CAD build for the part. Positions are in the model's coordinates, mm. A direction names the side the tool comes from. Give positions to 0.01 mm unless a question says otherwise; leave off trailing zeros. Order: outer loops, then holes, each group sorted by start corner. A loop starts at its lowest first (then second) coordinate and runs counter-clockwise, first axis right, second up.
from build123d import *

# Parameters (mm, degrees)
SALIENTE_EXTRUIR1_DEPTH    = 131.1
CROQUIS3_R                 = 1.1
CORTAR_EXTRUIR1_DEPTH      = 289.575068223
CROQUIS4_R                 = 10.7
CROQUIS4_R_2               = 5.07
CROQUIS4_W                 = 121.1
CROQUIS4_H                 = 75.8
CROQUIS4_W_2               = 1.6
CROQUIS4_H_2               = 10
CROQUIS4_W_3               = 10
CROQUIS4_H_3               = 10.6
CORTAR_EXTRUIR2_DEPTH      = 287.189954401
CROQUIS7_W                 = 1.36
CROQUIS7_H                 = 98
CROQUIS7_W_2               = 1.86
CROQUIS7_H_2               = 41.6
SALIENTE_EXTRUIR2_DEPTH    = 4.4
CROQUIS8_R                 = 2.27
CORTAR_EXTRUIR3_DEPTH      = 1.8
CORTAR_EXTRUIR4_START      = -1.8
CROQUIS9_R                 = 2.27
CORTAR_EXTRUIR4_DEPTH      = 1.8
CROQUIS10_R                = 11.9
CROQUIS10_R_2              = 10.7
CROQUIS10_W                = 12.4
CROQUIS10_H                = 13
CROQUIS10_W_2              = 10
CROQUIS10_H_2              = 10.6
SALIENTE_EXTRUIR4_DEPTH    = 8.6
REDONDEO2_R                = 1.28
CORTAR_EXTRUIR5_REACH      = 292.482
CORTAR_EXTRUIR5_END_RADIUS = 10.7
CROQUIS11_W                = 4
CROQUIS11_H                = 14
SALIENTE_EXTRUIR6_START    = 1
CROQUIS13_W                = 12.4
CROQUIS13_H                = 13
SALIENTE_EXTRUIR6_DEPTH    = 1
CROQUIS14_R                = 2.8
CROQUIS14_R_2              = 1.5
SALIENTE_EXTRUIR7_DEPTH    = 8.4
REDONDEO3_R                = 1.28
CROQUIS17_W                = 4.4
CROQUIS17_H                = 0.4
CORTAR_EXTRUIR6_DEPTH      = 285.106479335
REDONDEO4_R                = 1.6
CROQUIS19_R                = 1.12
SALIENTE_EXTRUIR8_DEPTH    = 8.6
REDONDEO5_R                = 1
CORTAR_EXTRUIR8_START      = -1.86
CROQUIS21_W                = 0.6
CROQUIS21_H                = 26
CORTAR_EXTRUIR8_DEPTH      = 1.86
CROQUIS23_W                = 121.1
CROQUIS23_H                = 0.1
CORTAR_EXTRUIR9_DEPTH      = 287.189954401
CORTAR_EXTRUIR10_DEPTH     = 286.758027009


with BuildPart() as part:
    # Croquis2 → Saliente-Extruir1 (new body)
    with BuildSketch(Plane(origin=(0, 0, 0), x_dir=(0, 0, -1), z_dir=(1, 0, 0))):
        with BuildLine():
            Line((37, 0), (37, -3.2))
            Line((37, -3.2), (8.4, -3.2))
            ThreePointArc((8.4, -3.2), (0.197561338, 0.197561338), (-3.2, 8.4))
            Line((-3.2, 8.4), (-3.2, 239.6))
            ThreePointArc((-3.2, 239.6), (0.197561338, 247.802438662), (8.4, 251.2))
            Line((8.4, 251.2), (37, 251.2))
            Line((37, 251.2), (37, 248))
            Line((37, 248), (8.4, 248))
            ThreePointArc((8.4, 248), (2.460303038, 245.539696962), (0, 239.6))
            Line((0, 239.6), (0, 8.4))
            ThreePointArc((0, 8.4), (2.460303038, 2.460303038), (8.4, 0))
            Line((8.4, 0), (37, 0))
        make_face()
    extrude(amount=SALIENTE_EXTRUIR1_DEPTH)

    # Croquis3 → Cortar-Extruir1 (cut, through all)
    with BuildSketch(Plane(origin=(0, 251.2, 0), x_dir=(1, 0, 0), z_dir=(0, 1, 0))):
        with Locations(Location((6.55, 22.7, 0), (0, 0, 270))):
            Circle(CROQUIS3_R)
        with Locations(Location((124.55, 22.7, 0), (0, 0, 270))):
            Circle(CROQUIS3_R)
    extrude(amount=-CORTAR_EXTRUIR1_DEPTH, mode=Mode.SUBTRACT)

    # Croquis4 → Cortar-Extruir2 (cut, through all)
    with BuildSketch(Plane.XY.offset(3.2)):
        with Locations((17, 79.6)):
            Circle(CROQUIS4_R)
        with Locations((65.55, 113.5)):
            Circle(CROQUIS4_R_2)
        with Locations((65.55, 196.1)):
            Rectangle(CROQUIS4_W, CROQUIS4_H)
        with Locations((9.2, 112)):
            Rectangle(CROQUIS4_W_2, CROQUIS4_H_2)
        with Locations((45.7, 91.4)):
            Rectangle(CROQUIS4_W_3, CROQUIS4_H_3)
        with Locations((5.8, 112)):
            Rectangle(CROQUIS4_W_2, CROQUIS4_H_2)
        with Locations((12.6, 112)):
            Rectangle(CROQUIS4_W_2, CROQUIS4_H_2)
        with Locations((16, 112)):
            Rectangle(CROQUIS4_W_2, CROQUIS4_H_2)
        with Locations((19.4, 112)):
            Rectangle(CROQUIS4_W_2, CROQUIS4_H_2)
        with Locations((22.8, 112)):
            Rectangle(CROQUIS4_W_2, CROQUIS4_H_2)
        with Locations((26.2, 112)):
            Rectangle(CROQUIS4_W_2, CROQUIS4_H_2)
        with Locations((29.6, 112)):
            Rectangle(CROQUIS4_W_2, CROQUIS4_H_2)
        with Locations((33, 112)):
            Rectangle(CROQUIS4_W_2, CROQUIS4_H_2)
        with Locations((36.4, 112)):
            Rectangle(CROQUIS4_W_2, CROQUIS4_H_2)
        with Locations((39.8, 112)):
            Rectangle(CROQUIS4_W_2, CROQUIS4_H_2)
        with Locations((43.2, 112)):
            Rectangle(CROQUIS4_W_2, CROQUIS4_H_2)
        with Locations((46.6, 112)):
            Rectangle(CROQUIS4_W_2, CROQUIS4_H_2)
        with Locations((50, 112)):
            Rectangle(CROQUIS4_W_2, CROQUIS4_H_2)
    extrude(amount=-CORTAR_EXTRUIR2_DEPTH, mode=Mode.SUBTRACT)

    # Croquis7 → Saliente-Extruir2 (add)
    with BuildSketch(Plane(origin=(0, 0, 0), x_dir=(-1, 0, 0), z_dir=(0, 0, -1))):
        Polygon((-127.46, 125.3), (-127.96, 125.3), (-127.96, 66.3), (-127.46, 66.3), (-126.1, 66.3), (-126.1, 125.3), align=None)
        with Locations((-126.78, 185)):
            Rectangle(CROQUIS7_W, CROQUIS7_H)
        with Locations((-4.32, 185)):
            Rectangle(CROQUIS7_W, CROQUIS7_H)
        Polygon((-3.64, 125.3), (-5, 125.3), (-5, 66.3), (-3.64, 66.3), (-3.14, 66.3), (-3.14, 125.3), align=None)
        with Locations((-127.03, 32.7)):
            Rectangle(CROQUIS7_W_2, CROQUIS7_H_2)
        with Locations((-4.07, 32.7)):
            Rectangle(CROQUIS7_W_2, CROQUIS7_H_2)
    extrude(amount=SALIENTE_EXTRUIR2_DEPTH)

    # Croquis8 → Cortar-Extruir3 (cut)
    with BuildSketch(Plane(origin=(0, 251.2, 0), x_dir=(1, 0, 0), z_dir=(0, 1, 0))):
        with Locations(Location((6.55, 22.7, 0), (0, 0, 270))):
            Circle(CROQUIS8_R)
        with Locations(Location((124.55, 22.7, 0), (0, 0, 270))):
            Circle(CROQUIS8_R)
    extrude(amount=-CORTAR_EXTRUIR3_DEPTH, mode=Mode.SUBTRACT)

    # Croquis9 → Cortar-Extruir4 (cut)
    with BuildSketch(Plane.XZ.offset(3.2).offset(CORTAR_EXTRUIR4_START)):
        with Locations(Location((124.55, -22.7, 0), (0, 0, 90))):
            Circle(CROQUIS9_R)
        with Locations(Location((6.55, -22.7, 0), (0, 0, 90))):
            Circle(CROQUIS9_R)
    extrude(amount=CORTAR_EXTRUIR4_DEPTH, mode=Mode.SUBTRACT)

    # Croquis10 → Saliente-Extruir4 (add)
    # profile 1 of 2: a face of its own
    with BuildSketch(Plane(origin=(0, 0, 0), x_dir=(-1, 0, 0), z_dir=(0, 0, -1))):
        with Locations(Location((-17, 79.6, 0), (0, 0, 180))):
            Circle(CROQUIS10_R)
        with Locations(Location((-17, 79.6, 0), (0, 0, 180))):
            Circle(CROQUIS10_R_2, mode=Mode.SUBTRACT)
    # profile 2 of 2: a face of its own
    with BuildSketch(Plane(origin=(0, 0, 0), x_dir=(-1, 0, 0), z_dir=(0, 0, -1))):
        with Locations((-45.7, 91.4)):
            Rectangle(CROQUIS10_W, CROQUIS10_H)
        with Locations((-45.7, 91.4)):
            Rectangle(CROQUIS10_W_2, CROQUIS10_H_2, mode=Mode.SUBTRACT)
    extrude(amount=SALIENTE_EXTRUIR4_DEPTH)

    # Redondeo2
    redondeo2_edges = [part.edges().sort_by_distance(p)[0] for p in [
        (40.7, 86.1, -2.7),
        (40.7, 96.7, -2.7),
        (50.7, 96.7, -2.7),
        (50.7, 86.1, -2.7),
    ]]
    fillet(redondeo2_edges, radius=REDONDEO2_R)

    # Cortar-Extruir5: up to this cylinder (the profile starts outside it)
    cortar_extruir5_end = Plane(origin=(17, 79.6, -4.3), z_dir=(0, 0, 1)) * Cylinder(CORTAR_EXTRUIR5_END_RADIUS, 607.364, mode=Mode.PRIVATE)
    # Croquis11 → Cortar-Extruir5 (cut, up to the surface)
    with BuildSketch(Plane.ZY.offset(10), mode=Mode.PRIVATE) as cortar_extruir5_sk1:
        with Locations((-4.3, 79.6)):
            Rectangle(CROQUIS11_W, CROQUIS11_H)
    cortar_extruir5_tool1 = extrude(cortar_extruir5_sk1.sketch, amount=-CORTAR_EXTRUIR5_REACH, mode=Mode.PRIVATE) - cortar_extruir5_end
    add(cortar_extruir5_tool1.solids().sort_by_distance((-10, 79.6, -4.3))[0], mode=Mode.SUBTRACT)

    # Croquis13 → Saliente-Extruir6 (add)
    with BuildSketch(Plane(origin=(0, 0, -8.6), x_dir=(-1, 0, 0), z_dir=(0, 0, -1)).offset(SALIENTE_EXTRUIR6_START)):
        with Locations((-45.7, 91.4)):
            Rectangle(CROQUIS13_W, CROQUIS13_H)
        with BuildLine():
            ThreePointArc((-49.42, 86.1), (-50.32509668, 86.47490332), (-50.7, 87.38))
            Line((-50.7, 87.38), (-50.7, 95.42))
            ThreePointArc((-50.7, 95.42), (-50.32509668, 96.32509668), (-49.42, 96.7))
            Line((-49.42, 96.7), (-41.98, 96.7))
            ThreePointArc((-41.98, 96.7), (-41.07490332, 96.32509668), (-40.7, 95.42))
            Line((-40.7, 95.42), (-40.7, 87.38))
            ThreePointArc((-40.7, 87.38), (-41.07490332, 86.47490332), (-41.98, 86.1))
            Line((-41.98, 86.1), (-49.42, 86.1))
        make_face(mode=Mode.SUBTRACT)
    extrude(amount=-SALIENTE_EXTRUIR6_DEPTH)

    # Croquis14 → Saliente-Extruir7 (add)
    with BuildSketch(Plane(origin=(0, 0, 0), x_dir=(-1, 0, 0), z_dir=(0, 0, -1))):
        with Locations(Location((-65.55, 88.8, 0), (0, 0, 180))):
            Circle(CROQUIS14_R)
        with Locations((-65.55, 88.8)):
            Circle(CROQUIS14_R_2, mode=Mode.SUBTRACT)
    extrude(amount=SALIENTE_EXTRUIR7_DEPTH)

    # Redondeo3
    redondeo3_edges = [part.edges().sort_by_distance(p)[0] for p in [
        (62.75, 88.8, 0),
    ]]
    fillet(redondeo3_edges, radius=REDONDEO3_R)

    # Croquis17 → Cortar-Extruir6 (cut, through all)
    with BuildSketch(Plane(origin=(127.46, 0, 0), x_dir=(0, 0, -1), z_dir=(1, 0, 0))):
        with Locations((2.2, 233.8)):
            Rectangle(CROQUIS17_W, CROQUIS17_H)
    extrude(amount=-CORTAR_EXTRUIR6_DEPTH, mode=Mode.SUBTRACT)

    # Redondeo4
    redondeo4_edges = [part.edges().sort_by_distance(p)[0] for p in [
        (51.9, 91.4, 0),
        (39.5, 91.4, 0),
    ]]
    fillet(redondeo4_edges, radius=REDONDEO4_R)

    # Croquis19 → Saliente-Extruir8 (add)
    with BuildSketch(Plane(origin=(0, 0, 0), x_dir=(-1, 0, 0), z_dir=(0, 0, -1))):
        with Locations((-17, 91.5)):
            Circle(CROQUIS19_R)
        with Locations((-17, 67.7)):
            Circle(CROQUIS19_R)
    extrude(amount=SALIENTE_EXTRUIR8_DEPTH)

    # Redondeo5
    redondeo5_edges = [part.edges().sort_by_distance(p)[0] for p in [
        (28.9, 79.6, 0),
    ]]
    fillet(redondeo5_edges, radius=REDONDEO5_R)

    # Croquis21 → Cortar-Extruir8 (cut)
    with BuildSketch(Plane(origin=(127.96, 0, 0), x_dir=(0, 0, -1), z_dir=(1, 0, 0)).offset(CORTAR_EXTRUIR8_START)):
        with Locations((4.1, 79.3)):
            Rectangle(CROQUIS21_W, CROQUIS21_H)
    extrude(amount=CORTAR_EXTRUIR8_DEPTH, mode=Mode.SUBTRACT)

    # Croquis23 → Cortar-Extruir9 (cut, through all)
    with BuildSketch(Plane.XY.offset(3.2)):
        with Locations((65.55, 158.15)):
            Rectangle(CROQUIS23_W, CROQUIS23_H)
    extrude(amount=-CORTAR_EXTRUIR9_DEPTH, mode=Mode.SUBTRACT)

    # Croquis24 → Cortar-Extruir10 (cut, through all)
    with BuildSketch(Plane(origin=(131.1, 0, 0), x_dir=(0, 0, -1), z_dir=(1, 0, 0))):
        with BuildLine():
            Line((37, 60.8), (37, 248))
            Line((37, 248), (8.4, 248))
            ThreePointArc((8.4, 248), (2.460303038, 245.539696962), (0, 239.6))
            Line((0, 239.6), (0, 60.8))
            Line((0, 60.8), (37, 60.8))
        make_face()
        with BuildLine():
            Line((37, 248), (37, 251.2))
            Line((37, 251.2), (8.4, 251.2))
            ThreePointArc((8.4, 251.2), (0.197561338, 247.802438662), (-3.2, 239.6))
            Line((-3.2, 239.6), (-3.2, 64.8))
            Line((-3.2, 64.8), (-1.6, 64.8))
            Line((-1.6, 64.8), (-1.6, 60.8))
            Line((-1.6, 60.8), (0, 60.8))
            Line((0, 60.8), (0, 239.6))
            ThreePointArc((0, 239.6), (2.460303038, 245.539696962), (8.4, 248))
            Line((8.4, 248), (37, 248))
        make_face()
    extrude(amount=-CORTAR_EXTRUIR10_DEPTH, mode=Mode.SUBTRACT)


solid = part.part
1. Mould opens along X. For faces 1 (the flat face through (127.96, 32, -2)), 2 (the flat face through (65, 35, 0)), 3 (the cylindrical face through (64.632, 2.526, -2.395)) say: released by +X, released by -X, zero draft, split by the parting line, or undercut.
2. Saw through at B-B on y = 51. Give the cut face in (x, z), plus the area to 3 significant figures.
3. Wall check: line 1 (X direction, y = -1.05, z = -22.7); line 2 (X direction, y = -2.75, z = -22.7); line 3 (Z direction, x = 52, y = 39.5). Give the ranges that are in metal, low to high.
4. Pin check, flat tips, straight feed: P1, Ø2, axis at x = 127, y = 28.5, coming from the -Z side; P2, Ø0.6, axis at x = 4, z = -2, coming from the -Y side; P3, Ø5, axis at x = 114, z = -22, coming from the +Y side; P4, Ø6, axis at y = 48, z = -10, coming from the -X side. Stop position of each tip, or through.
5. 3-axis set-ups, long thin cutter, end or side, ignore diameter. For faces 4 (the flat face through (8, -1.4, -23)), 5 (the flat face through (66, 63, 1.6)), 6 (the flat face through (3.14, 32, -2)), 7 (the flat face through (5, 32, -2)): which of +Z, -Z, +X, -X, +Y, -Y reach the whole face in a straight line?
6. Saw through at A-A on x = 115.5. Give the cut face in (y, z).
7. Saw through at C-C on z = -34. Give the cut face in (x, y), plus the area to 3 significant figures.
Reported:
1. face 1: released by +X
1. face 2: undercut
1. face 3: zero draft
2. outline: (0, 0) - (3.14, 0) - (3.14, -4.4) - (5, -4.4) - (5, 0) - (126.1, 0) - (126.1, -4.4) - (127.96, -4.4) - (127.96, 0) - (131.1, 0) - (131.1, 3.2) - (0, 3.2) - close
2. area: 436 mm2
3. line 1: x = 0 to 5.45, 7.65 to 123.45, 125.65 to 131.1
3. line 2: x = 0 to 4.28, 8.82 to 122.28, 126.82 to 131.1
3. line 3: z = 0 to 3.2
4. P1: stops at z = -4.4
4. P2: stops at y = -1.47
4. P3: stops at y = 0
4. P4: passes through
5. face 4: -Y
5. face 5: -Z, +X, -X, +Y
5. face 6: -Z, -X, +Y
5. face 7: -Z, +Y
6. outline: (-3.2, -37) - (0, -37) - (0, -8.4) arc R8.4 cw to (8.4, 0) - (60.8, 0) - (60.8, 1.6) - (64.8, 1.6) - (64.8, 3.2) - (8.4, 3.2) arc R11.6 ccw to (-3.2, -8.4) - close
7. outline: (0, -3.2) - (131.1, -3.2) - (131.1, 0) - (0, 0) - close
7. area: 420 mm2
